```python
from build123d import *

# Parameters (mm, degrees)
F0_R      = 12
F1_DEPTH  = 29.4
F0_R_2    = 44
F2_DEPTH  = 10.5
F5_W      = 14
F5_H      = 24
F6_DEPTH  = 16
F8_W      = 2
F8_H      = 7
F9_DEPTH  = 4
F10_W     = 7
F10_H     = 2
F11_DEPTH = 8


with BuildPart() as f1:
    # F0 (on Top) → F1 (new body)
    with BuildSketch(Plane.XY):
        Circle(F0_R)
    extrude(amount=-F1_DEPTH)

    # F0 (on Top) → F2 (join)
    with BuildSketch(Plane.XY):
        Circle(F0_R_2)
        Circle(F0_R, mode=Mode.SUBTRACT)
        Circle(F0_R)
    extrude(amount=F2_DEPTH)

    # F3 (on Front) → F4 (revolve)
    with BuildSketch(Plane.XZ):
        with BuildLine():
            Line((-49.5, 10.5), (0, 10.5))
            Line((0, 10.5), (0, 30.5))
            ThreePointArc((0, 30.5), (-26.4675851071, 24.7510231401), (-49.5, 10.5))
        make_face()
    revolve(axis=Axis((0, 0, 20.5), (0, 0, 1)))



with BuildPart() as f6:
    # F5 (on face) → F6 (new body)
    with BuildSketch(Plane(origin=(0, 0, -29.4), x_dir=(1, 0, 0), z_dir=(0, 0, -1))):
        with Locations((7, 0)):
            Rectangle(F5_W, F5_H)
    extrude(amount=F6_DEPTH)


with BuildPart() as f1_1:
    add(f1.part)

    add(f6.part)  # F7 merges F6
    # F7: F6 across face
    add(f6.part.mirror(Plane(origin=(0, 0, -37.4), x_dir=(0, -1, 0), z_dir=(-1, 0, 0))))

    # F8 (on face) → F9 (join)
    with BuildSketch(Plane(origin=(0, 0, -45.4), x_dir=(1, 0, 0), z_dir=(0, 0, -1))):
        with Locations((-1, 0)):
            Rectangle(F8_W, F8_H)
    extrude(amount=F9_DEPTH)

    # F10 (on face) → F11 (join)
    with BuildSketch(Plane.YZ):
        with Locations((0, -48.4)):
            Rectangle(F10_W, F10_H)
    extrude(amount=F11_DEPTH)


solid = f1_1.part
```
CAD build for the part. Positions are in the model's coordinates, mm. A direction names the side the tool comes from. Give positions to 0.01 mm unless a question says otherwise; leave off trailing zeros. Order: outer loops, then holes, each group sorted by start corner. A loop starts at its lowest first (then second) coordinate and runs counter-clockwise, first axis right, second up.
(1) Tool access for faces 1 (the flat face through (2, -3.5, -48)), 2 (the flat face through (-12.2, 0.8, -29.4)), 3 (the cylindrical face through (-9.538, -42.954, 5.176)), 4 (the cylindrical face through (-11.99, 0.53, -14.49)), 5 (the flat face through (-14, 0, -37)): list every direction of +Z, -Z, +X, -X, +Y, -Y with a clear straight run to the whole face (end or side of a thin tool).
(2) Drill centre lines: L1, parallel to Y at x = 1.5, z = -35.5; L2, parallel to X at y = -3, z = -43; L3, parallel to Z at x = -8.5, y = -11. Where is each one in solid material? Low to high.
(3) Mould opens along Z. For faces 6 (the flat face through (0, 12, -37)), 7 (the flat face through (33.23, 29.1, 10.5)), 8 (the flat face through (12.2, 0.8, -29.4)) say: released by +Z, released by -Z, zero draft, split by the parting line, or undercut.
(4) Saw through at A-A, the plane z = -44. Give the cut face in (x, y).
(5) Flat gauge pins, fed straight in: pin 1 (1 mm diameter, centred on y = -16.5, z = 15, fed in from -X); pin 2 (8 mm diameter, centred on x = -4, z = -35, fed in from -Y); pin 3 (4 mm diameter, centred on x = 8, y = 2.5, fed in from +Z). Where does each tip first touch, or does it go through?
Results found:
1. face 1: -Z, +X, -X, -Y
1. face 2: -X
1. face 3: -Z
1. face 4: none
1. face 5: -Z, -X, +Y, -Y
2. L1: y = -12 to 12
2. L2: x = -14 to 14
2. L3: z = -45.4 to -29.4, 0 to 28.66
3. face 6: zero draft
3. face 7: released by -Z
3. face 8: undercut
4. outline: (-14, -12) - (14, -12) - (14, 12) - (-14, 12) - close
5. pin 1: stops at x = -41.46
5. pin 2: stops at y = -12
5. pin 3: stops at z = 29.96
